Here's how the part is built. I have some questions about the finished solid (model axes, mm). Give positions to 0.01 mm unless a question says otherwise; leave off trailing zeros. Order: outer loops, then holes, each group sorted by start corner. A loop starts at its lowest first (then second) coordinate and runs counter-clockwise, first axis right, second up. Notation, with made-up numbers: M 38,-26 L 56,-26 A20 cw 56,-3 Z; hole C 28,68.5 d10. An arc over 180 degrees is marked long. One line per item, written item: value. Start each with the question number.
from build123d import *

# Parameters (mm, degrees)
F0_W     = 1450
F0_H     = 250
F1_DEPTH = 25
F2_R     = 1
F3_DEPTH = 25
F5_R     = 7.5
F6_DEPTH = 5
F7_R     = 5
F8_DEPTH = 5


with BuildPart() as f1:
    # F0 (on Top) → F1 (new body)
    with BuildSketch(Plane.XY):
        with Locations((0, -236.8958477461)):
            Rectangle(F0_W, F0_H)
    extrude(amount=F1_DEPTH)

    # F2 (on face) → F3 (join)
    with BuildSketch(Plane.XZ.offset(361.8958477461)):
        with Locations((-483.3333333333, 12.5)):
            Circle(F2_R)
        with Locations((-241.6666666667, 12.5)):
            Circle(F2_R)
        with Locations((0, 12.5)):
            Circle(F2_R)
        with Locations((241.6666666667, 12.5)):
            Circle(F2_R)
        with Locations((483.3333333333, 12.5)):
            Circle(F2_R)
    extrude(amount=F3_DEPTH)

    # F5 (on offset) → F6 (join)
    with BuildSketch(Plane.XZ.offset(386.8958477461)):
        with Locations((-483.3333333333, 12.5)):
            Circle(F5_R)
        with Locations((-241.6666666667, 12.5)):
            Circle(F5_R)
        with Locations((0, 12.5)):
            Circle(F5_R)
        with Locations((241.6666666667, 12.5)):
            Circle(F5_R)
        with Locations((483.3333333333, 12.5)):
            Circle(F5_R)
    extrude(amount=F6_DEPTH)

    # F7 (on face) → F8 (cut)
    with BuildSketch(Plane.XY.offset(25)):
        with Locations((-241.6666666667, -236.8958477461)):
            Circle(F7_R)
        with Locations((241.6666666667, -236.8958477461)):
            Circle(F7_R)
    extrude(amount=-F8_DEPTH, mode=Mode.SUBTRACT)


solid = f1.part
Item 1: Will these pins go through, and if not, where does the flat tip stop? P1, Ø6, axis at x = 154.5, z = 11.5, coming from the -Y side; P2, Ø3, axis at x = -242.5, y = -236.5, coming from the +Z side.
Item 2: We'd pull the mould along Y, two halves only. Please class faces 1 (the face through (-725, -239, 12)), 2 (the face through (-10, -111.896, 12)): +Y half, -Y half, draft (parallel to the pull), parting line (faces both ways), or undercut.
Item 3: Please list where this line runs through material, in increasing order: probe 1 along Y at (x, z) = (606, 19). Write a range as [from, to].
Item 4: I want a section at A-A on x = 28. Write out the boundary of the cut face in (y, z).
Answer below:
1. P1: stops at y = -361.9
1. P2: stops at z = 20
2. face 1: draft
2. face 2: +Y half
3. probe 1: y = [-361.9, -111.9]
4. outline: M -361.9,0 L -111.9,0 L -111.9,25 L -361.9,25 Z
